from build123d import *

# Parameters (mm, degrees)
SKETCH5_R          = 2.38125
CUT_EXTRUDE1_DEPTH = 24.019799782
SKETCH6_R          = 3.96875
CUT_EXTRUDE2_DEPTH = 0.9398


with BuildPart() as part:
    # Sketch3 → Revolve1 (revolve)
    with BuildSketch(Plane.XY):
        Polygon((13.312399842, 22.00099994), (16.639799842, 22.00099994), (16.639799842, 7.499999986), (18.039799836, 7.499999986), (23.019799782, 7.499999986), (23.019799782, 6.499999954), (20.019799813, 3.499999985), (16.119799866, 3.499999985), (16.119799866, 4.000000001), (13.639799746, 4.000000001), (13.639799746, 12.269749908), (13.312399842, 12.269749908), align=None)
    revolve(axis=Axis((0, 0, 0), (1, 0, 0)))

    # Sketch5 → Cut-Extrude1 (cut, through all)
    with BuildSketch(Plane(origin=(0, 0, 0), x_dir=(0, 0, -1), z_dir=(1, 0, 0))):
        with Locations((-14.928978871, 8.61924997)):
            Circle(SKETCH5_R)
        with Locations((0, 17.23849994)):
            Circle(SKETCH5_R)
        with Locations((14.928978871, 8.61924997)):
            Circle(SKETCH5_R)
        with Locations((14.928978871, -8.61924997)):
            Circle(SKETCH5_R)
        with Locations((0, -17.23849994)):
            Circle(SKETCH5_R)
        with Locations((-14.928978871, -8.61924997)):
            Circle(SKETCH5_R)
    extrude(amount=CUT_EXTRUDE1_DEPTH, mode=Mode.SUBTRACT)

    # Sketch6 → Cut-Extrude2 (cut)
    with BuildSketch(Plane(origin=(16.639799842, 0, 0), x_dir=(0, 0, -1), z_dir=(1, 0, 0))):
        with Locations((0, 17.23849994)):
            Circle(SKETCH6_R)
        with Locations((14.928978871, 8.61924997)):
            Circle(SKETCH6_R)
        with Locations((14.928978871, -8.61924997)):
            Circle(SKETCH6_R)
        with Locations((0, -17.23849994)):
            Circle(SKETCH6_R)
        with Locations((-14.928978871, -8.61924997)):
            Circle(SKETCH6_R)
        with Locations((-14.928978871, 8.61924997)):
            Circle(SKETCH6_R)
    extrude(amount=-CUT_EXTRUDE2_DEPTH, mode=Mode.SUBTRACT)


solid = part.part
Could you check a few things on this model? Use its own coordinates, in mm. A direction names the side the tool comes from. Round coordinates to 2 decimals unless told otherwise and drop trailing zeros. Write each loop counter-clockwise with the first axis right and the second up, starting at its lowest first coordinate (ties: lowest second). Pieces come first, ordered by that corner, then holes. Notation, with made-up numbers: (13, -30.75) -> (32, -30.75) arc R22 ccw to (32, -2.75) -> close; hole circle Ø6 at (-29, 5.25). An arc over 180 degrees is marked (long way). Use a Markdown table: item, result.
1. Please list where these lines run through material, in increasing order: probe 1 along Y at (x, z) = (14.5, -1); probe 2 along Z at (x, y) = (15.75, -7); probe 3 along X at (y, z) = (-16.5, 11).
Answer key:
| item | result |
|---|---|
| probe 1 | y = -21.98 to -19.4, -15.08 to -3.87, 3.87 to 15.08, 19.4 to 21.98 |
| probe 2 | z = -20.86 to -18.55, -11.31 to 11.31, 18.55 to 20.86 |
| probe 3 | x = 13.31 to 16.64 |
2. For pin 1 Ø1 at (x, z) = (17, 1) entering from +Y; pin 2 Ø2.5 at (y, z) = (-18.5, -1.5) entering from +X; pin 3 Ø2 at (x, y) = (15, -12) entering from +Z, each with a flat end and sliding along its axis, tell me the tip position at first contact or that it passes through.
Answer key:
| item | result |
|---|---|
| pin 1 | stops at y = 21.99 |
| pin 2 | stops at x = 15.7 |
| pin 3 | stops at z = 19.05 |
3. If we section it at B-B (x = 19): List the corners of the cut face in (y, z) for me, then the cut area to 3 significant figures.
Answer key:
| item | result |
|---|---|
| outline | circle Ø15 at (0, 0); hole circle Ø7 at (0, 0) |
| area | 138 mm^2 |
4. If we section it at D-D (x = 14.75): List the corners of the cut face in (y, z) for me.
Answer key:
| item | result |
|---|---|
| outline | circle Ø44 at (0, 0); hole circle Ø4.76 at (-17.24, 0); hole circle Ø4.76 at (-8.62, -14.93); hole circle Ø4.76 at (-8.62, 14.93); hole circle Ø8 at (0, 0); hole circle Ø4.76 at (8.62, -14.93); hole circle Ø4.76 at (8.62, 14.93); hole circle Ø4.76 at (17.24, 0) |
5. If we section it at C-C (z = 0): State how many separate pieces and enclosed holes the cut face has, then the cut area to 3 significant figures.
Answer key:
| item | result |
|---|---|
| separate pieces | 4 |
| enclosed holes | 0 |
| area | 119 mm^2 |
6. If we section it at A-A (y = 0): List the corners of the cut face in (x, z) for me.
Answer key:
| item | result |
|---|---|
| outline | (13.31, -22) -> (16.64, -22) -> (16.64, -7.5) -> (23.02, -7.5) -> (23.02, -6.5) -> (20.02, -3.5) -> (16.12, -3.5) -> (16.12, -4) -> (13.64, -4) -> (13.64, -12.27) -> (13.31, -12.27) -> close; (13.31, 12.27) -> (13.64, 12.27) -> (13.64, 4) -> (16.12, 4) -> (16.12, 3.5) -> (20.02, 3.5) -> (23.02, 6.5) -> (23.02, 7.5) -> (16.64, 7.5) -> (16.64, 22) -> (13.31, 22) -> close |
7. Which directions (+Z, -Z, +X, -X, +Y, -Y) give clear straight access to the entire face, cutting with the end or side of a thin tool? Please do faces 1 (the face through (16.64, 9, 0)), 2 (the face through (14.862, -0.521, 3.966)), 3 (the face through (14.49, -6.61, -16.21)).
Answer key:
| item | result |
|---|---|
| face 1 | +X |
| face 2 | -X |
| face 3 | +X, -X |
8. We'd pull the mould along Y, two halves only. Please class faces 4 (the face through (14.999, -16.216, 14.869)), 5 (the face through (15.7, -19, -2)), 6 (the face through (15.7, -11.2, 15)), 7 (the face through (23.02, -6, 3)): +Y half, -Y half, draft (parallel to the pull), parting line (faces both ways), or undercut.
Answer key:
| item | result |
|---|---|
| face 4 | parting line |
| face 5 | undercut |
| face 6 | undercut |
| face 7 | draft |
